The model under review builds one solid part; all positions refer to its coordinate system, in mm. A direction names the side the tool comes from. Give positions to 0.01 mm unless a question says otherwise; leave off trailing zeros. Order: outer loops, then holes, each group sorted by start corner. A loop starts at its lowest first (then second) coordinate and runs counter-clockwise, first axis right, second up.
```python
from build123d import *

# Parameters (mm, degrees)
SKETCH2_R           = 10
BOSS_EXTRUDE1_DEPTH = 15
SKETCH4_R           = 10
BOSS_EXTRUDE2_DEPTH = 50
SKETCH5_W           = 30
SKETCH5_H           = 72.699493752
CUT_EXTRUDE1_DEPTH  = 25


with BuildPart() as part:
    # Sketch2 → Boss-Extrude1 (new body)
    with BuildSketch(Plane(origin=(0, 0, 0), x_dir=(1, 0, 0), z_dir=(0, 1, 0))):
        with BuildLine():
            Line((-35.258358851, 25), (44.741641149, 25))
            ThreePointArc((44.741641149, 25), (69.741641149, 0), (44.741641149, -25))
            Line((44.741641149, -25), (-35.258358851, -25))
            ThreePointArc((-35.258358851, -25), (-60.258358851, 0), (-35.258358851, 25))
        make_face()
        with Locations((-35.258358851, 0)):
            Circle(SKETCH2_R, mode=Mode.SUBTRACT)
        with Locations((44.741641149, 0)):
            Circle(SKETCH2_R, mode=Mode.SUBTRACT)
    extrude(amount=BOSS_EXTRUDE1_DEPTH)

    # Sketch4 → Boss-Extrude2 (add)
    with BuildSketch(Plane.XY.offset(25)):
        with BuildLine():
            Line((-20, 67.699493752), (-20, 15))
            Line((-20, 15), (20, 15))
            Line((20, 15), (20, 67.699493752))
            ThreePointArc((20, 67.699493752), (0, 87.699493752), (-20, 67.699493752))
        make_face()
        with Locations((0, 67.699493752)):
            Circle(SKETCH4_R, mode=Mode.SUBTRACT)
    extrude(amount=-BOSS_EXTRUDE2_DEPTH)

    # Sketch5 → Cut-Extrude1 (cut, symmetric)
    with BuildSketch(Plane(origin=(0, 0, 0), x_dir=(0, 0, -1), z_dir=(1, 0, 0))):
        with Locations((0, 51.349746876)):
            Rectangle(SKETCH5_W, SKETCH5_H)
    extrude(amount=CUT_EXTRUDE1_DEPTH, both=True, mode=Mode.SUBTRACT)


solid = part.part
```
Item 1: Take a section at C-C (x = 0). Give the boundary of the cut face in (y, z).
Values found:
outline: (0, -25) - (57.7, -25) - (57.7, -15) - (15, -15) - (15, 15) - (57.7, 15) - (57.7, 25) - (0, 25) - close; (77.7, -25) - (87.7, -25) - (87.7, -15) - (77.7, -15) - close; (77.7, 15) - (87.7, 15) - (87.7, 25) - (77.7, 25) - close
Item 2: Take a section at D-D (y = 64.5). Give the boundary of the cut face in (x, z), and give its area (3 significant figures).
Values found:
outline: (-20, -25) - (-9.47, -25) - (-9.47, -15) - (-20, -15) - close; (-20, 15) - (-9.47, 15) - (-9.47, 25) - (-20, 25) - close; (9.47, -25) - (20, -25) - (20, -15) - (9.47, -15) - close; (9.47, 15) - (20, 15) - (20, 25) - (9.47, 25) - close
area: 421 mm2
Item 3: Draft analysis for pull direction Y (two halves, no side actions). For faces 5 (the cylindrical face through (-2.168, 57.937, 20.07)), 6 (the flat face through (20, 41, -20)), 7 (the flat face through (6, 0, 0)), 8 (the cylindrical face through (0.44, 87.695, 20.07)), state which applies: released by +Y, released by -Y, zero draft, split by the parting line, or undercut.
Values found:
face 5: undercut
face 6: zero draft
face 7: released by -Y
face 8: released by +Y
Item 4: Clearance check with flat-ended pins moving along their axes: pin 1 Ø8 at (y, z) = (30.5, -13) entering from +X; pin 2 Ø3 at (y, z) = (38, -17.5) entering from -X; pin 3 Ø1.5 at (x, z) = (-16, 16.5) entering from +Y. State where each tip first meets the part, or that it passes through.
Values found:
pin 1: stops at x = 20
pin 2: stops at x = -20
pin 3: stops at y = 80.64
Item 5: For faces 1 (the cylindrical face through (-2.168, 57.937, -19.93)), 2 (the flat face through (-20, 42, 20)), 3 (the flat face through (0, 43, 15)), 4 (the flat face through (20, 41, 20)), list the 3-axis set-ups (+Z, -Z, +X, -X, +Y, -Y) from which the entire face can be reached by the end or side of a thin tool; tool diameter is ignored.
Values found:
face 1: +Z, -Z
face 2: +Z, -Z, -X, +Y
face 3: +X, -X, +Y
face 4: +Z, -Z, +X, +Y
Item 6: Take a section at B-B (y = 24.5). Give the boundary of the cut face in (x, z).
Values found:
outline: (-20, -25) - (20, -25) - (20, -15) - (-20, -15) - close; (-20, 15) - (20, 15) - (20, 25) - (-20, 25) - close
Item 7: Take a section at A-A (z = 0). Give the boundary of the cut face in (x, y).
Values found:
outline: (-60.26, 0) - (-45.26, 0) - (-45.26, 15) - (-60.26, 15) - close; (-25.26, 0) - (34.74, 0) - (34.74, 15) - (-25.26, 15) - close; (54.74, 0) - (69.74, 0) - (69.74, 15) - (54.74, 15) - close
Item 8: For line 1 (X direction, y = 4.75, z = 0); line 2 (Z direction, x = -4, y = 31); line 3 (Z direction, x = -35, y = 12.5), list the stretches that pass through material, from the lowest coordinate up.
Values found:
line 1: x = -60.26 to -45.26, -25.26 to 34.74, 54.74 to 69.74
line 2: z = -25 to -15, 15 to 25
line 3: z = -25 to -10, 10 to 25
